Work out the finished part from the listing and answer in its coordinate system (mm). Face numbers are marked on the shaded views. A direction names the side the tool comes from. Round coordinates to 2 decimals unless told otherwise and drop trailing zeros. Order: outer loops, then holes, each group sorted by start corner. A loop starts at its lowest first (then second) coordinate and runs counter-clockwise, first axis right, second up.
from build123d import *

# Parameters (mm, degrees)
F0_R     = 12.7
F0_R_2   = 9.525
F1_DEPTH = 38.1
F2_W     = 38.1
F2_H     = 38.1
F2_R     = 9.525
F3_DEPTH = 6.35
F4_R     = 12.7
F4_R_2   = 9.525
F5_DEPTH = 38.1


with BuildPart() as f1:
    # F0 (on Top) → F1 (new body)
    with BuildSketch(Plane.XY):
        Circle(F0_R)
        Circle(F0_R_2, mode=Mode.SUBTRACT)
    extrude(amount=F1_DEPTH)

    # F2 (on Top) → F3 (join)
    with BuildSketch(Plane.XY):
        Rectangle(F2_W, F2_H)
        Circle(F2_R, mode=Mode.SUBTRACT)
    extrude(amount=F3_DEPTH)

    # F4 (on face) → F5 (join)
    with BuildSketch(Plane(origin=(0, 0, 0), x_dir=(1, 0, 0), z_dir=(0, 0, -1))):
        Circle(F4_R)
        Circle(F4_R_2, mode=Mode.SUBTRACT)
    extrude(amount=F5_DEPTH)


solid = f1.part
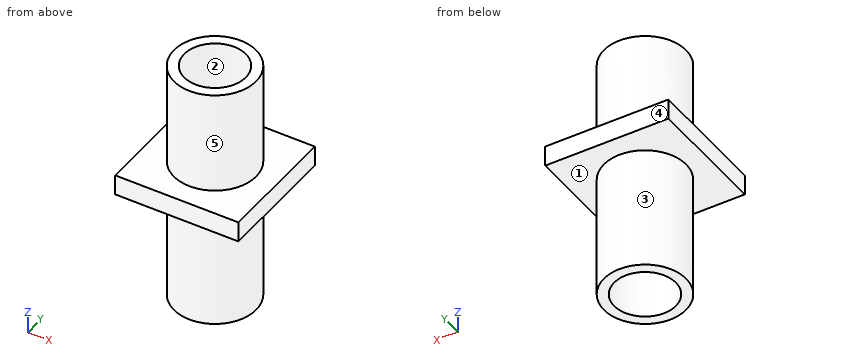
Item 1: Find section C-C (z = 30). Write down the section's boundary in (x, y) (3 decimals).
Item 2: For a pull along X with two mould halves and no side action, classify the marked faces 1, 2 and 3 as released by +X, released by -X, zero draft, split by the parting line, or undercut.
Item 3: Find the intervals of material crossed by line 1 along X through (y, z) = (0, 13) (3 decimals); line 2 along Y through (x, z) = (0, 3) (3 decimals), in increasing order.
Item 4: Find section A-A (y = 0). Write down the section's boundary in (x, z) (3 decimals), plus the area to 3 significant figures.
Item 5: Given pin 1 (2 mm diameter, centred on x = -13, y = 14, fed in from -Z); pin 2 (1.5 mm diameter, centred on x = 4, z = -18, fed in from -Y); pin 3 (2 mm diameter, centred on x = -9, z = -4, fed in from -Y), each flat-ended and moving along its own axis, determine where each tip first touches the part or whether it passes through.
Item 6: Find section D-D (y = 11). Write down the section's boundary in (x, z).
Item 7: A tool of negligible diameter and unlimited length cuts with its end or side. For the marked faces 4 and 5, from which of +Z, -Z, +X, -X, +Y, -Y can it reach the whole face along a straight path? Write none if from no direction.
Model answer:
1. outline: circle Ø25.4 at (0, 0); hole circle Ø19.05 at (0, 0)
2. face 1: zero draft
2. face 2: undercut
2. face 3: split by the parting line
3. line 1: x = -12.7 to -9.525, 9.525 to 12.7
3. line 2: y = -19.05 to -9.525, 9.525 to 19.05
4. outline: (-19.05, 0) - (-12.7, 0) - (-12.7, -38.1) - (-9.525, -38.1) - (-9.525, 38.1) - (-12.7, 38.1) - (-12.7, 6.35) - (-19.05, 6.35) - close; (9.525, -38.1) - (12.7, -38.1) - (12.7, 0) - (19.05, 0) - (19.05, 6.35) - (12.7, 6.35) - (12.7, 38.1) - (9.525, 38.1) - close
4. area: 565 mm2
5. pin 1: stops at z = 0
5. pin 2: stops at y = -12.28
5. pin 3: stops at y = -9.86
6. outline: (-19.05, 0) - (-6.35, 0) - (-6.35, -38.1) - (6.35, -38.1) - (6.35, 0) - (19.05, 0) - (19.05, 6.35) - (6.35, 6.35) - (6.35, 38.1) - (-6.35, 38.1) - (-6.35, 6.35) - (-19.05, 6.35) - close
7. face 4: +Z, -Z, +X, -X, +Y
7. face 5: +Z
